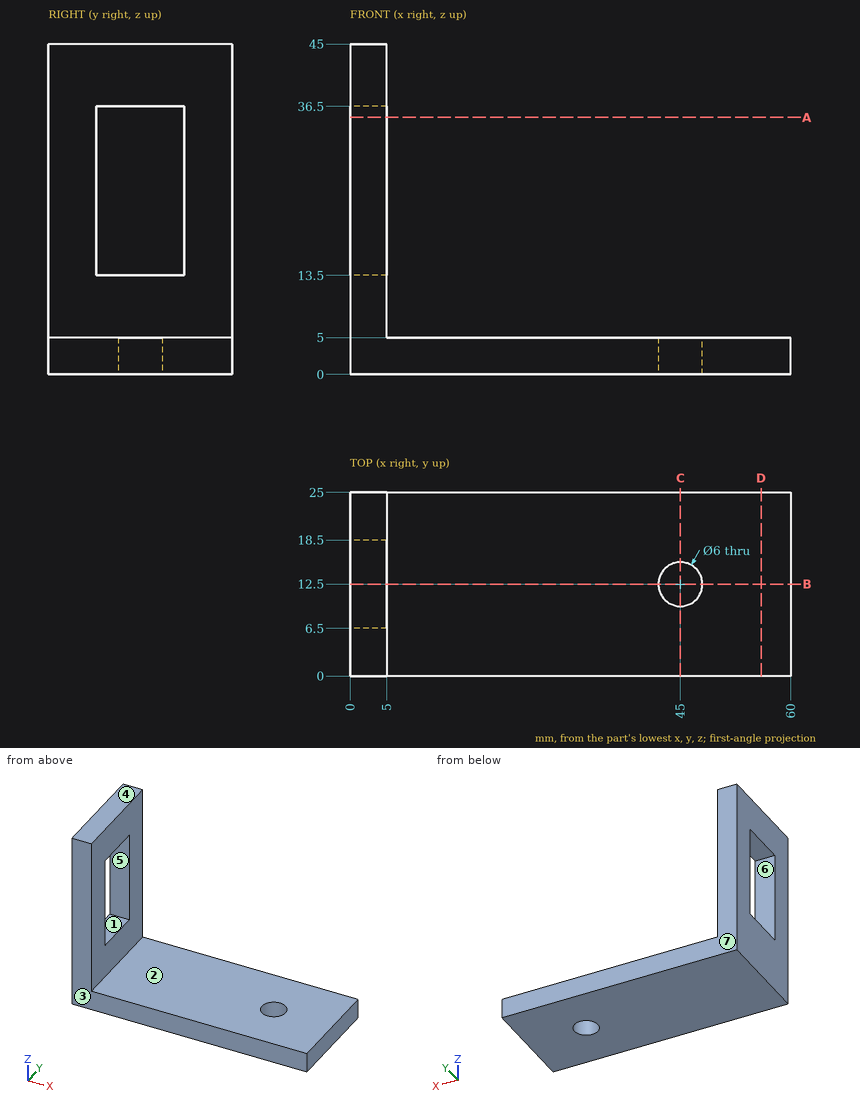
Geometry: see drawing. Coordinates: mm, zero at the bounding-box minimum. A direction names the side the tool comes from. Give positions to 0.01 mm unless a question says otherwise; leave off trailing zeros. Loops run counter-clockwise (first coordinate to the right, second up) from the corner with the lowest first, then second, coordinate; pieces in that order, holes last. Notation, with made-up numbers: (65, 83) -> (113, 83) arc R16 cw to (113, 110) -> close; hole circle Ø7 at (-21, 87). An arc over 180 degrees is marked (long way). Answer as a JSON object with one key per item and string values. Group by question number.
Item 1: Pull-direction query (Y, two-part tool) for the marked faces 4, 5, 6 and 7; classes: released by +Y, released by -Y, zero draft, split by the parting line, or undercut.
Item 2: Cut plane A-A, the plane z = 35. Return the cut outline in (x, y).
Item 3: Cut plane B-B, the plane y = 12.5. Return the cut outline in (x, z).
Item 4: Cut plane D-D, the plane x = 56. Return the cut outline in (y, z), and give its area (3 significant figures).
Item 5: Line query: probe 1 along Y at (x, z) = (45, 3.7); probe 2 along Z at (x, y) = (38.5, 17.5). Output: solid intervals per line, ascending.
Item 6: Cut plane C-C, the plane x = 45. Return the cut outline in (y, z), and give its area (3 significant figures).
Item 7: Reachability of the marked faces 1, 2 and 3 from +Z, -Z, +X, -X, +Y, -Y: full face, straight path, thin tool, end or side. Return the list, or none.
Item 8: Pin query (flat end, axial travel): P1, Ø1.5, axis at x = 50, y = 7, coming from the -Z side; P2, Ø7.5, axis at x = 24, y = 10.5, coming from the +Z side; P3, Ø10, axis at y = 16.5, z = 25.5, coming from the +X side; P4, Ø7.5, axis at y = 13, z = 32.5, coming from the +X side. Return the tip coordinate at first contact, or that it passes through.
Checks:
{
 "1": {"face 4": "zero draft", "face 5": "undercut", "face 6": "undercut", "face 7": "released by +Y"},
 "2": {"outline": "(0, 0) -> (5, 0) -> (5, 6.5) -> (0, 6.5) -> close; (0, 18.5) -> (5, 18.5) -> (5, 25) -> (0, 25) -> close"},
 "3": {"outline": "(0, 0) -> (42, 0) -> (42, 5) -> (5, 5) -> (5, 13.5) -> (0, 13.5) -> close; (0, 36.5) -> (5, 36.5) -> (5, 45) -> (0, 45) -> close; (48, 0) -> (60, 0) -> (60, 5) -> (48, 5) -> close"},
 "4": {"outline": "(0, 0) -> (25, 0) -> (25, 5) -> (0, 5) -> close", "area": "125 mm²"},
 "5": {"probe 1": "y = 0 to 9.5, 15.5 to 25", "probe 2": "z = 0 to 5"},
 "6": {"outline": "(0, 0) -> (9.5, 0) -> (9.5, 5) -> (0, 5) -> close; (15.5, 0) -> (25, 0) -> (25, 5) -> (15.5, 5) -> close", "area": "95.0 mm²"},
 "7": {"face 1": "+X, -X", "face 2": "+Z, +X, +Y, -Y", "face 3": "+Z, -Z, +X, -X, -Y"},
 "8": {"P1": "stops at z = 0", "P2": "stops at z = 5", "P3": "stops at x = 5", "P4": "passes through"}
}
